Can you work these out from the model? Positions are in its coordinate system, mm. Face numbers are marked on the shaded views. A direction names the side the tool comes from. Round coordinates to 2 decimals unless told otherwise and drop trailing zeros. Order: outer loops, then holes, each group sorted by start corner. A loop starts at its lowest first (then second) coordinate and runs counter-clockwise, first axis right, second up.
from build123d import *

# Parameters (mm, degrees)
SKETCH_W        = 40
SKETCH_H        = 25
PAD_DEPTH       = 15
SKETCH001_R     = 3.25
POCKET_DEPTH    = 40.001
SKETCH002_R     = 3.25
POCKET001_DEPTH = 25.001
SKETCH003_W     = 5.5
SKETCH003_H     = 10.5
POCKET002_DEPTH = 15.001
FILLET_R        = 2


with BuildPart() as part:
    # Sketch → Pad (new body)
    with BuildSketch(Plane.XY):
        with Locations((20, 12.5)):
            Rectangle(SKETCH_W, SKETCH_H)
    extrude(amount=PAD_DEPTH)

    # Sketch001 (on Face2 of Pad) → Pocket (cut, through all)
    with BuildSketch(Plane.YZ.offset(40)):
        with Locations((12.5, 7.5)):
            Circle(SKETCH001_R)
    extrude(amount=-POCKET_DEPTH, mode=Mode.SUBTRACT)

    # Sketch002 (on Face1 of Pocket) → Pocket001 (cut, through all)
    with BuildSketch(Plane.XZ):
        with Locations((20, 7.5)):
            Circle(SKETCH002_R)
    extrude(amount=-POCKET001_DEPTH, mode=Mode.SUBTRACT)

    # Sketch003 (on Face4 of Pocket001) → Pocket002 (cut, through all)
    with BuildSketch(Plane.XY.offset(15)):
        with Locations((7.75, 12.5)):
            Rectangle(SKETCH003_W, SKETCH003_H)
        with Locations((32.25, 12.5)):
            Rectangle(SKETCH003_W, SKETCH003_H)
    extrude(amount=-POCKET002_DEPTH, mode=Mode.SUBTRACT)

    # Fillet
    fillet_edges = [part.edges().sort_by_distance(p)[0] for p in [
        (20, 0, 15),
        (20, 0, 0),
        (20, 25, 15),
        (20, 25, 0),
    ]]
    fillet(fillet_edges, radius=FILLET_R)


solid = part.part
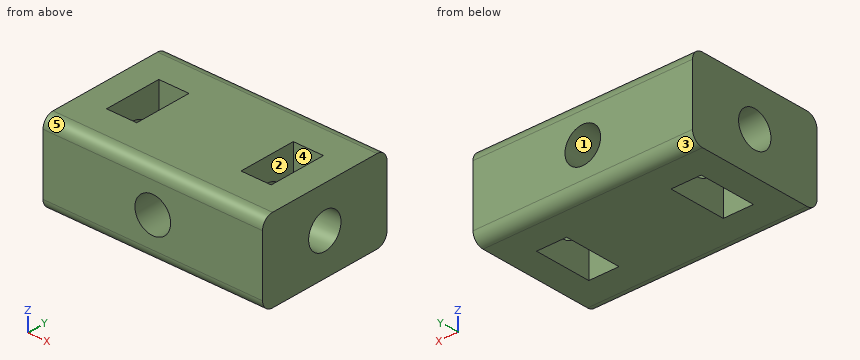
(1) I want a section at B-B, the plane z = 7.5. Give the number of separate pieces and of enclosed holes in the cut face, plus the area to 3 significant figures.
(2) I'm going to push a flat-ended pin straight in: pin 1 Ø4 at (x, z) = (20, 7.5) entering from -Y. Where does the tip first touch, or does it pass through?
(3) Please list where these lines run through material, in increasing order: probe 1 along Y at (x, z) = (24.25, 7.5); probe 2 along Z at (x, y) = (38.15, 12.5); probe 3 along X at (y, z) = (12.25, 12).
(4) On a 3-axis mill with a long thin cutter (end or side, diameter ignored), from which of +Z, -Z, +X, -X, +Y, -Y can I reach the whole of each face in a straight line? I mean the marked faces 4 and 5. Say none if no direction works.
(5) I want a section at C-C, the plane x = 6.5. List the corners of the cut face in (y, z) for me.
(6) I want a section at A-A, the plane y = 8.5. List the corners of the cut face in (x, z) for me, plus the area to 3 significant figures.
(7) I want a section at D-D, the plane x = 26.5. List the corners of the cut face in (y, z) for me, plus the area to 3 significant figures.
(8) If we mould it in two halves opening along Y, with no side actions, what happens to the marked faces 1, 2 and 3? For each: pulls with the +Y half, pulls with the -Y half, needs draft (parallel to the pull), parting line crosses it, or undercut.
Ans:
1. separate pieces: 4
1. enclosed holes: 0
1. area: 576 mm2
2. pin 1: passes through
3. probe 1: y = 0 to 9.25, 15.75 to 25
3. probe 2: z = 0 to 4.25, 10.75 to 15
3. probe 3: x = 0 to 5, 10.5 to 29.5, 35 to 40
4. face 4: +Z, -Z
4. face 5: +Z, +X, -X, -Y
5. outline: (0, 2) arc R2 ccw to (2, 0) - (7.25, 0) - (7.25, 15) - (2, 15) arc R2 ccw to (0, 13) - close; (17.75, 0) - (23, 0) arc R2 ccw to (25, 2) - (25, 13) arc R2 ccw to (23, 15) - (17.75, 15) - close
6. outline: (0, 0) - (5, 0) - (5, 15) - (0, 15) - close; (10.5, 0) - (29.5, 0) - (29.5, 15) - (10.5, 15) - close; (35, 0) - (40, 0) - (40, 15) - (35, 15) - close; hole circle Ø6.5 at (20, 7.5)
6. area: 402 mm2
7. outline: (0, 2) arc R2 ccw to (2, 0) - (23, 0) arc R2 ccw to (25, 2) - (25, 13) arc R2 ccw to (23, 15) - (2, 15) arc R2 ccw to (0, 13) - close; hole circle Ø6.5 at (12.5, 7.5)
7. area: 338 mm2
8. face 1: needs draft
8. face 2: undercut
8. face 3: pulls with the +Y half
